Autodesk Inventor part; units mm, degrees
ref_plane "YZ Plane" through (0, 0, 0) normal (1, 0, 0) x (0, 1, 0)
ref_plane "XZ Plane" through (0, 0, 0) normal (0, 1, 0) x (-1, 0, 0)
ref_plane "XY Plane" through (0, 0, 0) normal (0, 0, 1) x (1, 0, 0)
sketch "Sketch1" plane through (0, 0, 0) normal (0, 0, 1) x (1, 0, 0)
  line L0 (0, 0) -> (63.5, 0)
  line L1 (63.5, 0) -> (63.5, 38.1)
  line L2 (63.5, 38.1) -> (0, 38.1)
  line L3 (0, 38.1) -> (0, 0)
  dimension "d0" = 63.5
  dimension "d1" = 38.1
extrude "Extrusion1" add sketch "Sketch1" along normal blind 6.35
sketch "Sketch2" plane through (0, 0, 6.35) normal (0, 0, 1) x (1, 0, 0)
  line L0 (0, 38.1) -> (0, 0)
  line L1 (0, 19.05) -> (12.7, 19.05)
  line L2 (63.5, 0) -> (63.5, 38.1)
  line L3 (63.5, 19.05) -> (50.8, 19.05)
  line L4 (63.5, 19.05) -> (76.2, 19.05) construction
  dimension "d4" = 12.7
  dimension "d5" = 12.7
  dimension "d6" = 180
hole "Hole1" at (12.7, 19.05, 6.35) at (50.8, 19.05, 6.35) direction (0, 0, -1) diameter 7.62 depth 25.4 tip angle 118
properties part number "RelicArmSpacer"
Read the model definition and answer for the solid it produces. Units are mm, in the model's axes. Coordinates: 2 decimals unless noted, no trailing zeros. Loops run counter-clockwise (first coordinate to the right, second up) from the corner with the lowest first, then second, coordinate; pieces in that order, holes last.
(1) A flat-ended cylindrical pin translates along its axis: pin 1 Ø3 at (x, y) = (18, 19) entering from -Z. Find the tip coordinate at first contact, or state that the pin passes through.
Solution:
pin 1: stops at z = 0
(2) The mould has two halves that part along Y. Classify faces 1 (the face through (32, 38.1, 3)), 2 (the face through (16.08, 17.29, 3.13)), 3 (the face through (31, 19, 0)): released by +Y, released by -Y, zero draft, split by the parting line, or undercut.
Solution:
face 1: released by +Y
face 2: undercut
face 3: zero draft
(3) The part is cut by section C-C (z = 0.75). Determine the outline of the cut face in (x, y), and give its area (3 significant figures).
Solution:
outline: (0, 0) - (63.5, 0) - (63.5, 38.1) - (0, 38.1) - close; hole circle Ø7.62 at (12.7, 19.05); hole circle Ø7.62 at (50.8, 19.05)
area: 2,330 mm2
(4) The part is cut by section A-A (y = 19.05). Determine the outline of the cut face in (x, z).
Solution:
outline: (0, 0) - (8.89, 0) - (8.89, 6.35) - (0, 6.35) - close; (16.51, 0) - (46.99, 0) - (46.99, 6.35) - (16.51, 6.35) - close; (54.61, 0) - (63.5, 0) - (63.5, 6.35) - (54.61, 6.35) - close
(5) Consider line 1 along X through (y, z) = (19.05, 4); line 2 along Y through (x, z) = (12.7, 5.25); line 3 along X through (y, z) = (21, 4). Determine where each line is inside the solid, lowest interval first.
Solution:
line 1: x = 0 to 8.89, 16.51 to 46.99, 54.61 to 63.5
line 2: y = 0 to 15.24, 22.86 to 38.1
line 3: x = 0 to 9.43, 15.97 to 47.53, 54.07 to 63.5
(6) The part is cut by section B-B (x = 50.8). Determine the outline of the cut face in (y, z).
Solution:
outline: (0, 0) - (15.24, 0) - (15.24, 6.35) - (0, 6.35) - close; (22.86, 0) - (38.1, 0) - (38.1, 6.35) - (22.86, 6.35) - close
